Geometry check sheet. Reference: the model listing, model coordinates, mm. Face numbers are marked on the shaded views. A direction names the side the tool comes from. Coordinates: 2 decimals unless noted, no trailing zeros. Write each loop counter-clockwise with the first axis right and the second up, starting at its lowest first coordinate (ties: lowest second). Pieces come first, ordered by that corner, then holes.
from build123d import *

# Parameters (mm, degrees)
EXTRUDE_START                      = 0.2
EXTRUDE_1_DEPTH                    = 5.1
SKETCH_7_W                         = 0.3
SKETCH_7_H                         = 0.2
EXTRUDE_4_DEPTH                    = 11.5
SKETCH_8_W                         = 1
SKETCH_8_H                         = 2
CUT_EXTRUDE_5_DEPTH                = 6.03
CUT_EXTRUDE_1_DEPTH                = 9.2
EXTRUDE_2_DEPTH                    = 3.8
SKETCH_4_W                         = 5.63
SKETCH_4_H                         = 1
CUT_EXTRUDE_2_DEPTH                = 3.8
CUT_EXTRUDE_3_REACH                = 17.116
CHAMFER_1_SIZE                     = 0.5
CUT_EXTRUDE_6_REACH                = 16.052
SKETCH_9_W                         = 0.7
SKETCH_9_H                         = 1
SWEEP_START                        = 0.95
SWEEP_1_DEPTH                      = 0.64
CHAMFER_2_SIZE                     = 0.2
PATTERN_LINEAR_2_COUNT             = 2
PATTERN_LINEAR_2_PITCH             = 2.54
PATTERN_LINEAR_1_COUNT             = 2
PATTERN_LINEAR_1_PITCH             = 2.54
CHAMFER_2_OF_PATTERN_LINEAR_1_SIZE = 0.2


# Read off the part's stored shape, not the designer's step: По траектории1
with BuildPart() as part:
    # Эскиз1 → Бобышка-Вытянуть1 (new body)
    with BuildSketch(Plane.XY.offset(EXTRUDE_START)):
        Polygon((-3.015, 0.55), (3.015, 0.55), (3.015, -1.45), (3.815, -1.45), (3.815, -12.95), (-3.815, -12.95), (-3.815, -1.45), (-3.015, -1.45), align=None)
    extrude(amount=EXTRUDE_1_DEPTH)

    # Эскиз7 → Бобышка-Вытянуть4 (add)
    with BuildSketch(Plane.XZ.offset(12.95)):
        with Locations((2.265, 0.1)):
            Rectangle(SKETCH_7_W, SKETCH_7_H)
        with Locations((-2.265, 0.1)):
            Rectangle(SKETCH_7_W, SKETCH_7_H)
    extrude(amount=-EXTRUDE_4_DEPTH)

    # Эскиз8 → Вырез-Вытянуть5 (cut)
    with BuildSketch(Plane(origin=(3.015, 0, 0), x_dir=(0, 0, -1), z_dir=(1, 0, 0))):
        with Locations((-0.7, -0.45)):
            Rectangle(SKETCH_8_W, SKETCH_8_H)
        Polygon((-4.2, -1.45), (-5.3, -1.45), (-5.3, 0.55), (-3.9, 0.55), (-3.9, -0.45), (-4.2, -0.45), align=None)
    extrude(amount=-CUT_EXTRUDE_5_DEPTH, mode=Mode.SUBTRACT)

    # Эскиз2 → Вырез-Вытянуть1 (cut)
    with BuildSketch(Plane.XZ.offset(12.95)):
        Polygon((-2.815, 4.3), (-2.815, 1.2), (-0.6, 1.2), (-0.6, 0.2), (0.6, 0.2), (0.6, 1.2), (2.815, 1.2), (2.815, 4.3), (1.5, 4.3), (1.5, 5.3), (-1.5, 5.3), (-1.5, 4.3), align=None)
    extrude(amount=-CUT_EXTRUDE_1_DEPTH, mode=Mode.SUBTRACT)

    # Эскиз3 → Бобышка-Вытянуть2 (add)
    with BuildSketch(Plane.XZ.offset(12.95)):
        Polygon((-3.815, 5.3), (-3.815, 6.8), (3.815, 6.8), (3.815, 5.3), (2.815, 5.3), (2.815, 5.8), (-2.815, 5.8), (-2.815, 5.3), align=None)
    extrude(amount=-EXTRUDE_2_DEPTH)

    # Эскиз4 → Вырез-Вытянуть2 (cut)
    with BuildSketch(Plane.XZ.offset(12.95)):
        with Locations((0, 4.8)):
            Rectangle(SKETCH_4_W, SKETCH_4_H)
    extrude(amount=-CUT_EXTRUDE_2_DEPTH, mode=Mode.SUBTRACT)

    # Эскиз5 → Вырез-Вытянуть3 (cut, up to next)
    with BuildSketch(Plane.XY.offset(6.8), mode=Mode.PRIVATE) as cut_extrude_3_sk1:
        with BuildLine():
            Line((2.815, -9.15), (2.815, -10.95))
            ThreePointArc((2.815, -10.95), (2.668553391, -11.303553391), (2.315, -11.45))
            Line((2.315, -11.45), (-2.315, -11.45))
            ThreePointArc((-2.315, -11.45), (-2.668553391, -11.303553391), (-2.815, -10.95))
            Line((-2.815, -10.95), (-2.815, -9.15))
            Line((-2.815, -9.15), (2.815, -9.15))
        make_face()
    cut_extrude_3_tool1 = extrude(cut_extrude_3_sk1.sketch, amount=-CUT_EXTRUDE_3_REACH, mode=Mode.PRIVATE) & part.part
    add(cut_extrude_3_tool1.solids().sort_by_distance((0, -10.291324, 6.8))[0], mode=Mode.SUBTRACT)

    # Фаска1
    chamfer_1_edges = [part.edges().sort_by_distance(p)[0] for p in [
        (0, -12.95, 5.8),
        (-2.1575, -9.15, 4.3),
        (2.1575, -9.15, 4.3),
        (-2.815, -12.95, 3.5),
        (-1.7075, -12.95, 1.2),
        (1.7075, -12.95, 1.2),
        (2.815, -12.95, 3.5),
    ]]
    chamfer(chamfer_1_edges, length=CHAMFER_1_SIZE)

    # Эскиз9 → Вырез-Вытянуть6 (cut, up to next)
    with BuildSketch(Plane.XY.offset(3.9), mode=Mode.PRIVATE) as cut_extrude_6_sk1:
        with Locations((1.275, 0.05)):
            Rectangle(SKETCH_9_W, SKETCH_9_H)
    cut_extrude_6_tool1 = extrude(cut_extrude_6_sk1.sketch, amount=-CUT_EXTRUDE_6_REACH, mode=Mode.PRIVATE) & part.part
    cut_extrude_6 = cut_extrude_6_tool1.solids().sort_by_distance((1.275, 0.05, 3.9))[0]
    add(cut_extrude_6, mode=Mode.SUBTRACT)

    # По траектории1 outline → По траектории1 (add)
    with BuildSketch(Plane.YZ.offset(SWEEP_START)):
        with BuildLine():
            Line((-3.75, 2.43), (-3.75, 3.07))
            add(Edge.make_bspline(
                [(-3.75, 3.07), (-4.166666667, 3.07), (-4.583333333, 3.07), (-6.516666667, 3.07), (-8.033333333, 3.07), (-9.55, 3.07)],
                knots=[0.623544277, 0.623544277, 0.623544277, 0.623544277, 0.704676976, 0.704676976, 1, 1, 1, 1], degree=3))
            Line((-9.55, 3.07), (-9.55, 2.43))
            Line((-9.55, 2.43), (-3.75, 2.43))
        make_face()
        with BuildLine():
            Line((0.32, -3.3), (0.32, 2.3))
            add(Edge.make_bspline(
                [(0.32, 2.3), (0.32, 2.499654349), (0.23877091, 2.700173533), (0.022322877, 2.916621566), (-0.064240468, 2.973940923), (-0.250203983, 3.050392149), (-0.370157621, 3.069944018), (-0.45, 3.07)],
                knots=[0.363474491, 0.363474491, 0.363474491, 0.363474491, 0.386414221, 0.386414221, 0.397884087, 0.397884087, 0.409353952, 0.409353952, 0.409353952, 0.409353952], degree=3))
            Line((-0.45, 3.07), (-0.45, 2.43))
            ThreePointArc((-0.45, 2.43), (-0.358076118, 2.391923882), (-0.32, 2.3))
            Line((-0.32, 2.3), (-0.32, -3.3))
            Line((-0.32, -3.3), (0.32, -3.3))
        make_face()
    sweep_1 = extrude(amount=SWEEP_1_DEPTH)

    # Фаска2
    chamfer_2_edges = [part.edges().sort_by_distance(p)[0] for p in [
        (1.27, -9.55, 3.07),
        (1.59, -9.55, 2.75),
        (1.27, -9.55, 2.43),
        (0.95, -9.55, 2.75),
        (1.27, -0.32, -3.3),
        (1.59, 0, -3.3),
        (1.27, 0.32, -3.3),
        (0.95, 0, -3.3),
    ]]
    chamfer(chamfer_2_edges, length=CHAMFER_2_SIZE)

    # Линейный массив2: Вырез-Вытянуть6 ×2
    with Locations(*[(-i * PATTERN_LINEAR_2_PITCH, 0, 0) for i in range(1, PATTERN_LINEAR_2_COUNT)]):
        add(cut_extrude_6, mode=Mode.SUBTRACT)

    # Линейный массив1: По траектории1 ×2
    with Locations(*[(-i * PATTERN_LINEAR_1_PITCH, 0, 0) for i in range(1, PATTERN_LINEAR_1_COUNT)]):
        add(sweep_1)

    # Фаска2 of Линейный массив1
    chamfer_2_of_pattern_linear_1_edges = [part.edges().sort_by_distance(p)[0] for p in [
        (-1.27, -9.55, 3.07),
        (-0.95, -9.55, 2.75),
        (-1.27, -9.55, 2.43),
        (-1.59, -9.55, 2.75),
        (-1.27, -0.32, -3.3),
        (-0.95, 0, -3.3),
        (-1.27, 0.32, -3.3),
        (-1.59, 0, -3.3),
    ]]
    chamfer(chamfer_2_of_pattern_linear_1_edges, length=CHAMFER_2_OF_PATTERN_LINEAR_1_SIZE)


solid = part.part
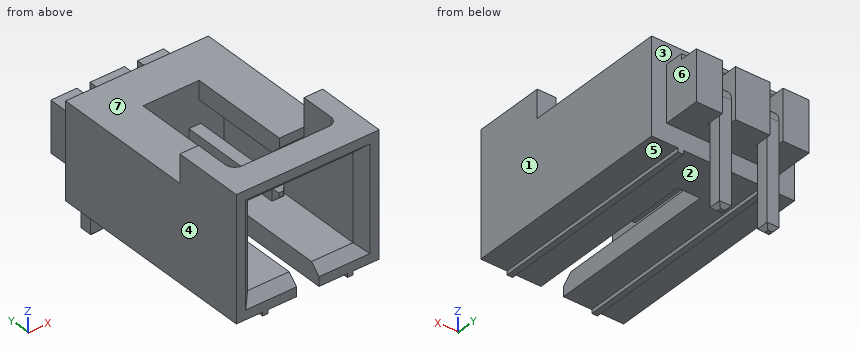
1. Sectioned sample at A-A, the plane z = -0.5. Record the boundary of the cut face in (x, y), and give its area (3 significant figures).
Computed values:
outline: (-1.59, -0.32) - (-0.95, -0.32) - (-0.95, 0.32) - (-1.59, 0.32) - close; (0.95, -0.32) - (1.59, -0.32) - (1.59, 0.32) - (0.95, 0.32) - close
area: 0.819 mm2
2. Sectioned sample at C-C, the plane y = -10.75. Record the boundary of the cut face in (x, z) (3 decimals).
Computed values:
outline: (-3.815, 0.2) - (-2.415, 0.2) - (-2.415, 0) - (-2.115, 0) - (-2.115, 0.2) - (-0.6, 0.2) - (-0.6, 1.2) - (-2.815, 1.2) - (-2.815, 6.8) - (-3.815, 6.8) - close; (0.6, 0.2) - (2.115, 0.2) - (2.115, 0) - (2.415, 0) - (2.415, 0.2) - (3.815, 0.2) - (3.815, 6.8) - (2.815, 6.8) - (2.815, 1.2) - (0.6, 1.2) - close
3. Sectioned sample at D-D, the plane y = -2. Record the boundary of the cut face in (x, z) (3 decimals), and give its area (3 significant figures).
Computed values:
outline: (-3.815, 0.2) - (-2.415, 0.2) - (-2.415, 0) - (-2.115, 0) - (-2.115, 0.2) - (2.115, 0.2) - (2.115, 0) - (2.415, 0) - (2.415, 0.2) - (3.815, 0.2) - (3.815, 5.3) - (-3.815, 5.3) - close
area: 39.0 mm2
4. Access from +Z, -Z, +X, -X, +Y, -Y to the whole of each face (thin tool, end or side, straight path). Record for the marked faces 5, 6 and 7.
Computed values:
face 5: -Z, +X, +Y, -Y
face 6: +Z, -Z, +X, +Y
face 7: +Z, +X, -X, +Y
5. Draft check along X on the marked faces 1, 2, 3 and 4. Enter one of: released by +X, released by -X, zero draft, split by the parting line, or undercut.
Computed values:
face 1: released by +X
face 2: undercut
face 3: zero draft
face 4: released by -X
6. Thickness scan on line 1 along X through (y, z) = (-4.75, 2.75) (3 decimals); line 2 along Z through (x, y) = (-2.25, -6); line 3 along X through (y, z) = (-7, 3.25) (3 decimals). Record the ranges inside material, lowest first.
Computed values:
line 1: x = -3.815 to -2.815, -1.59 to -0.95, 0.95 to 1.59, 2.815 to 3.815
line 2: z = 0 to 1.2, 4.3 to 5.3
line 3: x = -3.815 to -2.815, 2.815 to 3.815
7. Sectioned sample at B-B, the plane x = 0.75. Record the boundary of the cut face in (y, z), and give its area (3 significant figures).
Computed values:
outline: (-12.95, 0.2) - (-1.45, 0.2) - (-1.45, 1.2) - (0.55, 1.2) - (0.55, 3.9) - (-0.45, 3.9) - (-0.45, 4.2) - (-1.45, 4.2) - (-1.45, 5.3) - (-3.75, 5.3) - (-3.75, 1.2) - (-12.45, 1.2) - (-12.95, 0.7) - close; (-12.95, 6.3) - (-12.45, 5.8) - (-11.45, 5.8) - (-11.45, 6.8) - (-12.95, 6.8) - close
area: 27.9 mm2
8. Gauge pin test, flat ends, axial feed: pin 1 Ø1.3 at (x, y) = (-1, -7) entering from -Z; pin 2 Ø2.5 at (x, y) = (1.5, -7.5) entering from +Z; pin 3 Ø1.1 at (y, z) = (0, 2) entering from +X (3 decimals). Record the tip position at first contact, or that the pin passes through.
Computed values:
pin 1: stops at z = 0.2
pin 2: stops at z = 5.3
pin 3: stops at x = 3.015
